Read the model definition and answer for the solid it produces. Units are mm, in the model's axes. A direction names the side the tool comes from. Coordinates: 2 decimals unless noted, no trailing zeros. Loops run counter-clockwise (first coordinate to the right, second up) from the corner with the lowest first, then second, coordinate; pieces in that order, holes last. Notation, with made-up numbers: M 5,-39.5 L 23,-39.5 A24 cw 23,-26.5 Z; hole C 3,7 d2. An arc over 180 degrees is marked long. Use one line per item in the form item = value. Start each with the question number.
1. Find the intervals of material crossed by probe 1 along Y at (x, z) = (36.7, 3); probe 2 along Z at (x, y) = (37.45, 39); probe 3 along Y at (x, z) = (37.85, 38), in increasing order. Write a range as [from, to].
2. The part is cut by section C-C (y = 14). Give the vertices of the cut face in (x, z).
3. The part is cut by section A-A (z = 7.5). Give the vertices of the cut face in (x, y), plus the area to 3 significant figures.
4. The part is cut by section D-D (z = 43.5). Give the vertices of the cut face in (x, y).
5. Flat-ended cylindrical pins translate along their axes: pin 1 (1.5 mm diameter, centred on x = 37, y = 34, fed in from -Z); pin 2 (0.9 mm diameter, centred on x = 38, z = 9.5, fed in from +Y); pin 3 (0.9 mm diameter, centred on x = 37, y = -49.5, fed in from +Z). Find the tip coordinate at first contact, or state that the pin passes through.
6. For a pull along Y with two mould halves and no side action, classify faces 6 (the flat face through (38, 8, 10)), 7 (the flat face through (38, -50, 60)), 8 (the flat face through (38, 65.84, 65)), 9 (the flat face through (38, -48.16, 10)) as released by +Y, released by -Y, zero draft, split by the parting line, or undercut.
7. A tool of negligible diameter and unlimited length cuts with its end or side. For faces 1 (the flat face through (38, -50, 20)), 2 (the flat face through (38, -48.16, 65)), 3 (the flat face through (38, -50, 45)), 4 (the flat face through (38, 67, 45)), 5 (the flat face through (38, 65.84, 10)), from which of +Z, -Z, +X, -X, +Y, -Y can it reach the whole face along a straight path? Write none if from no direction.
8. The part is cut by section B-B (x = 37.6). Give the vertices of the cut face in (y, z).
Autodesk Fusion 360 part; units mm, degrees
sketch "Sketch1" plane through (0, 0, 0) normal (0, 0, 1) x (1, 0, 0)
  line L0 (36.0863, 68.8405) -> (39.0863, 68.8405)
  line L1 (39.0863, 68.8405) -> (39.0863, -51.1595)
  line L2 (39.0863, -51.1595) -> (36.0863, -51.1595)
  line L3 (36.0863, -51.1595) -> (36.0863, 68.8405)
  dimension "d1" = 3
  dimension "d2" = 120
extrude "Extrude1" add sketch "Sketch1" along normal blind 70
sketch "Sketch2" plane through (36.0863, 0, 0) normal (-1, 0, 0) x (0, -1, 0)
  line L0 (-68.8405, 0) -> (51.1595, 0)
  line L1 (51.1595, 0) -> (51.1595, 70)
  line L2 (51.1595, 70) -> (-68.8405, 70)
  line L3 (-68.8405, 70) -> (-68.8405, 0)
  line L4 (-58.8405, 0) -> (41.1595, 0)
  line L5 (41.1595, 0) -> (41.1595, 10)
  line L6 (41.1595, 10) -> (-58.8405, 10)
  line L7 (-58.8405, 10) -> (-58.8405, 0)
  dimension "d5" = 10
  dimension "d6" = 100
  dimension "d7" = 10
extrude "Extrude2" cut sketch "Sketch2" against normal blind 15 contours L0 L4 L5 L6 L7
sketch "Sketch3" plane through (36.0863, 0, 0) normal (-1, 0, 0) x (0, -1, 0)
  line L0 (41.1595, 10) -> (41.1595, 0)
  line L1 (41.1595, 0) -> (51.1595, 0)
  line L2 (51.1595, 0) -> (51.1595, 70)
  line L3 (51.1595, 70) -> (-68.8405, 70)
  line L4 (-68.8405, 70) -> (-68.8405, 0)
  line L5 (-68.8405, 0) -> (-58.8405, 0)
  line L6 (-58.8405, 0) -> (-58.8405, 10)
  line L7 (-58.8405, 10) -> (41.1595, 10)
  line L8 (-81.9379, 60) -> (81.0278, 60) construction
  line L9 (-84.1729, 45) -> (76.1854, 45) construction
  line L10 (-82.6829, 35) -> (77.4892, 35) construction
  line L11 (-85.6629, 20) -> (78.0479, 20) construction
  line L12 (-65.8405, 82.86) -> (-65.8405, -11.3972) construction
  line L13 (48.1595, 79.5603) -> (48.1595, -14.1231) construction
  line L14 (-65.8405, 60) -> (-65.8405, 45) construction
  line L15 (-65.8405, 45) -> (-68.8405, 45) construction
  line L16 (-68.8405, 35) -> (-65.8405, 35) construction
  line L17 (-65.8405, 35) -> (-65.8405, 20) construction
  line L18 (-65.8405, 20) -> (-68.8405, 20) construction
  line L19 (51.1595, 20) -> (48.1595, 20) construction
  line L20 (48.1595, 20) -> (48.1595, 35) construction
  line L21 (48.1595, 35) -> (51.1595, 35) construction
  line L22 (51.1595, 35) -> (51.1595, 20) construction
  line L23 (51.1595, 45) -> (48.1595, 45) construction
  line L24 (48.1595, 60) -> (51.1595, 60) construction
  line L25 (51.1595, 60) -> (51.1595, 45) construction
  line L26 (-65.8405, 45) -> (-68.8405, 45)
  line L27 (-65.8405, 60) -> (-68.8405, 60)
  line L28 (-68.8405, 60) -> (-68.8405, 70)
  line L29 (-68.8405, 70) -> (-65.8405, 70)
  line L30 (-65.8405, 70) -> (-65.8405, 60)
  line L31 (-65.8405, 35) -> (-68.8405, 35)
  line L32 (-68.8405, 35) -> (-68.8405, 45)
  line L33 (-68.8405, 45) -> (-65.8405, 45)
  line L34 (-65.8405, 45) -> (-65.8405, 35)
  line L35 (-65.8405, 0) -> (-68.8405, 0)
  line L36 (-68.8405, 0) -> (-68.8405, 20)
  line L37 (-68.8405, 20) -> (-65.8405, 20)
  line L38 (-65.8405, 20) -> (-65.8405, 0)
  line L39 (51.1595, 0) -> (48.1595, 0)
  line L40 (48.1595, 0) -> (48.1595, 20)
  line L41 (48.1595, 20) -> (51.1595, 20)
  line L42 (51.1595, 20) -> (51.1595, 0)
  line L43 (51.1595, 35) -> (48.1595, 35)
  line L44 (48.1595, 35) -> (48.1595, 45)
  line L45 (48.1595, 45) -> (51.1595, 45)
  line L46 (51.1595, 45) -> (51.1595, 35)
  line L47 (51.1595, 60) -> (48.1595, 60)
  line L48 (48.1595, 60) -> (48.1595, 70)
  line L49 (48.1595, 70) -> (51.1595, 70)
  line L50 (51.1595, 70) -> (51.1595, 60)
  dimension "d10" = 10
  dimension "d11" = 15
  dimension "d12" = 10
  dimension "d13" = 15
  dimension "d14" = 3
  dimension "d15" = 3
extrude "Extrude3" cut sketch "Sketch3" against normal blind 30 contours L1 L2 L39 L40 L41 L42 | L4 L5 L35 L36 L37 L38 | L2 L43 L44 L45 L46 | L4 L26 L31 L32 L33 L34 | L2 L3 L47 L48 L49 L50 | L3 L4 L27 L28 L29 L30
Computed values:
q1.probe_1 = [-48.16, -41.16], [58.84, 65.84]
q1.probe_2 = [10, 70]
q1.probe_3 = [-48.16, 65.84]
q2.outline = M 36.09,10 L 39.09,10 L 39.09,70 L 36.09,70 Z
q3.outline = M 36.09,-48.16 L 39.09,-48.16 L 39.09,-41.16 L 36.09,-41.16 Z; M 36.09,58.84 L 39.09,58.84 L 39.09,65.84 L 36.09,65.84 Z
q3.area = 42.0 mm²
q4.outline = M 36.09,-48.16 L 39.09,-48.16 L 39.09,65.84 L 36.09,65.84 Z
q5.pin_1 = 10
q5.pin_2 = 65.84
q5.pin_3 = 60
q6.face_6 = undercut
q6.face_7 = zero draft
q6.face_8 = released by +Y
q6.face_9 = released by -Y
q7.face_1 = -Z, +X, -X, -Y
q7.face_2 = +Z, +X, -X, -Y
q7.face_3 = +X, -X, -Y
q7.face_4 = +X, -X, +Y
q7.face_5 = -Z, +X, -X, +Y
q8.outline = M -51.16,20 L -48.16,20 L -48.16,0 L -41.16,0 L -41.16,10 L 58.84,10 L 58.84,0 L 65.84,0 L 65.84,20 L 68.84,20 L 68.84,35 L 65.84,35 L 65.84,45 L 68.84,45 L 68.84,60 L 65.84,60 L 65.84,70 L -48.16,70 L -48.16,60 L -51.16,60 L -51.16,45 L -48.16,45 L -48.16,35 L -51.16,35 Z
